```python
from build123d import *

# Parameters (mm, degrees)
BOSS_EXTRUDE1_DEPTH = 6.35
SKETCH2_R           = 5
CUT_EXTRUDE1_DEPTH  = 6.35
SKETCH3_R           = 11
CUT_EXTRUDE2_DEPTH  = 7.3500001
SKETCH4_W           = 15
SKETCH4_H           = 110
BOSS_EXTRUDE3_DEPTH = 6.35
SKETCH5_W           = 15
SKETCH5_H           = 50
BOSS_EXTRUDE4_DEPTH = 6.35


with BuildPart() as part:
    # Sketch1 → Boss-Extrude1 (new body)
    with BuildSketch(Plane(origin=(0, 0, 0), x_dir=(1, 0, 0), z_dir=(0, 1, 0))):
        with BuildLine():
            Line((0, 110), (0, 0))
            add(Edge.make_bspline(
                [(0, 0), (67.941176471, 0), (105, 25)],
                knots=[1.570796327, 1.570796327, 1.570796327, 2.564661308, 2.564661308, 2.564661308], degree=2, weights=[1, 0.879049073, 1]))
            Line((105, 25), (105, 85))
            add(Edge.make_bspline(
                [(105, 85), (67.941176471, 110), (0, 110)],
                knots=[3.718523999, 3.718523999, 3.718523999, 4.71238898, 4.71238898, 4.71238898], degree=2, weights=[1, 0.879049073, 1]))
        make_face()
    extrude(amount=BOSS_EXTRUDE1_DEPTH)

    # Sketch2 → Cut-Extrude1 (cut)
    with BuildSketch(Plane(origin=(0, 0, 0), x_dir=(1, 0, 0), z_dir=(0, 1, 0))):
        with Locations((95, 67.5)):
            Circle(SKETCH2_R)
        with Locations((95, 42.5)):
            Circle(SKETCH2_R)
    extrude(amount=CUT_EXTRUDE1_DEPTH, mode=Mode.SUBTRACT)

    # Sketch3 → Cut-Extrude2 (cut, through all)
    with BuildSketch(Plane(origin=(0, 0, 0), x_dir=(1, 0, 0), z_dir=(0, 1, 0))):
        with Locations((65, 55)):
            Circle(SKETCH3_R)
    extrude(amount=CUT_EXTRUDE2_DEPTH, mode=Mode.SUBTRACT)

    # Sketch4 → Boss-Extrude3 (add)
    with BuildSketch(Plane(origin=(0, 0, 0), x_dir=(1, 0, 0), z_dir=(0, 1, 0))):
        with Locations((-7.5, 55)):
            Rectangle(SKETCH4_W, SKETCH4_H)
    extrude(amount=BOSS_EXTRUDE3_DEPTH)

    # Sketch5 → Boss-Extrude4 (add)
    with BuildSketch(Plane(origin=(0, 0, 0), x_dir=(1, 0, 0), z_dir=(0, 1, 0))):
        with Locations((-7.5, 135)):
            Rectangle(SKETCH5_W, SKETCH5_H)
    extrude(amount=BOSS_EXTRUDE4_DEPTH)


solid = part.part
```
Design review of the part built by this model. Coordinates are the model's own, in mm. Coordinates: 2 decimals unless noted, no trailing zeros. Loops run counter-clockwise (first coordinate to the right, second up) from the corner with the lowest first, then second, coordinate; pieces in that order, holes last. Notation, with made-up numbers: M 50.25,34.25 L 104.25,34.25 A22 ccw 104.25,56.25 Z; hole C -13.5,-11.75 d9. An arc over 180 degrees is marked long. One line per question, with ' | ' between items.
(1) For pin 1 Ø9 at (x, z) = (95, -42.5) entering from +Y, flat-tipped, find the tip position at first contact; note if it passes through.
Filled in:
pin 1: passes through
(2) We need section A-A (z = -55). Give the boundary of the cut face in (x, y).
Filled in:
outline: M -15,0 L 54,0 L 54,6.35 L -15,6.35 Z; M 76,0 L 105,0 L 105,6.35 L 76,6.35 Z
(3) Wall thickness on probe 1 along Z at (x, y) = (95, 4.75); probe 2 along Z at (x, y) = (96.5, 4); probe 3 along X at (y, z) = (5.25, -68.5): over which ranges is each line inside the solid? List them lowest first.
Filled in:
probe 1: z = -90.85 to -72.5, -62.5 to -47.5, -37.5 to -19.15 | probe 2: z = -90.07 to -72.27, -62.73 to -47.27, -37.73 to -19.93 | probe 3: x = -15 to 90.1, 99.9 to 105
(4) Draft analysis for pull direction Z (two halves, no side actions). For faces 1 (the face through (-8, 3, 0)), 2 (the face through (56.89, 3.13, -62.43)), 3 (the face through (99.77, 3.13, -69)), 4 (the face through (0, 3, -135)), state which applies: released by +Z, released by -Z, zero draft, split by the parting line, or undercut.
Filled in:
face 1: released by +Z | face 2: undercut | face 3: undercut | face 4: zero draft
(5) We need section D-D (z = -148.5). Give the boundary of the cut face in (x, y), and give its area (4 significant figures).
Filled in:
outline: M -15,0 L 0,0 L 0,6.35 L -15,6.35 Z | area: 95.25 mm^2
(6) We need section B-B (y = 3.5). Count the separate pieces of the cut face and the enclosed holes in it, and give its area (3 significant figures).
Filled in:
separate pieces: 1 | enclosed holes: 3 | area: 11,900 mm^2
